from build123d import *

# Parameters (mm, degrees)
F0_R         = 12.0396
F0_R_2       = 10.7696
F1_DEPTH     = 12.065
F2_R         = 20.6121
F3_DEPTH     = 4.445
F5_DEPTH     = 16.511
F6_S5_R      = 12.0396
F6_T6_DEPTH  = 7
F6_S11_R     = 12.0396
F6_T12_DEPTH = 7
F6_S17_R     = 12.0396
F6_T18_DEPTH = 7
F6_S23_R     = 12.0396
F6_T24_DEPTH = 7
F7_W         = 10.7836972851
F7_H         = 1.905
F7_W_2       = 1.905
F7_H_2       = 10.8237928489
F7_W_3       = 10.1713027149
F7_H_3       = 10.1312071511
F8_DEPTH     = 2.54


# Not quite as in the source:
# - a fillet or chamfer that OpenCascade refuses, or shapes differently, is made with other operations: its cross-section is extruded or revolved along the edge and cut away or added


with BuildPart() as f1:
    # F0 (on Top) → F1 (new body)
    with BuildSketch(Plane.XY):
        with Locations((-31.5266512334, -46.8901731074)):
            Circle(F0_R)
        with Locations((-31.5266512334, -46.8901731074)):
            Circle(F0_R_2, mode=Mode.SUBTRACT)
    extrude(amount=F1_DEPTH)

    # F2 (on face) → F3 (join)
    with BuildSketch(Plane.XY.offset(12.065)):
        with Locations((-31.5266512334, -46.8901731074)):
            Circle(F2_R)
    extrude(amount=F3_DEPTH)

    # F4 (on face) → F5 (cut, through all)
    with BuildSketch(Plane.XY.offset(16.51)):
        with BuildLine():
            ThreePointArc((-31.7884928641, -33.1131611233), (-30.2443193797, -32.4476041714), (-29.6082253852, -30.8910624162))
            ThreePointArc((-29.6082253852, -30.8910624162), (-33.4171313906, -29.3345206609), (-31.7884928641, -33.1131611233))
        make_face()
        with BuildLine():
            ThreePointArc((-13.3019866134, -46.5860989557), (-15.5486867731, -44.3606454902), (-17.7526926267, -46.6283895083))
            ThreePointArc((-17.7526926267, -46.6283895083), (-15.5063943113, -48.8115524211), (-13.3019866134, -46.5860989557))
        make_face()
        with BuildLine():
            ThreePointArc((-28.9935999678, -62.8892183723), (-29.6606432601, -61.3004657527), (-31.2619205449, -60.6640753873))
            ThreePointArc((-31.2619205449, -60.6640753873), (-32.777664533, -64.4779709918), (-28.9935999678, -62.8892183723))
        make_face()
        with BuildLine():
            ThreePointArc((-45.3002079959, -47.1942472591), (-45.3003084592, -47.1731010282), (-45.3006098402, -47.1519567065))
            ThreePointArc((-45.3006098402, -47.1519567065), (-49.7512153901, -47.21539349), (-45.3002079959, -47.1942472591))
        make_face()
    extrude(amount=-F5_DEPTH, mode=Mode.SUBTRACT)

    # F6: chamfer of 1.905 on 4 edges, made by hand


with BuildPart() as f6_tool2:
    # F6_s3 → F6_t4 (revolve)
    with BuildSketch(Plane.XZ.offset(62.8892183723)):
        Polygon((-27.0885999678, 12.065), (-28.9935999678, 13.97), (-28.9935999678, 12.065), align=None)
    revolve(axis=Axis((-31.2191538966, -62.8892183723, 12.065), (0, 0, 1)))

    # F6_s5 → F6_t6 (cut, symmetric)
    with BuildSketch(Plane.XY.offset(13)):
        with Locations((-31.5266512334, -46.8901731074)):
            Circle(F6_S5_R)
    extrude(amount=F6_T6_DEPTH, both=True, mode=Mode.SUBTRACT)


with BuildPart() as f1_1:
    add(f1.part)

    # F6_t1: cut F6_tool2
    add(f6_tool2.part, mode=Mode.SUBTRACT)


with BuildPart() as f6_tool8:
    # F6_s9 → F6_t10 (revolve)
    with BuildSketch(Plane.XZ.offset(46.5860989557)):
        Polygon((-11.3969866134, 12.065), (-13.3019866134, 13.97), (-13.3019866134, 12.065), align=None)
    revolve(axis=Axis((-15.5275405422, -46.5860989557, 12.065), (0, 0, 1)))

    # F6_s11 → F6_t12 (cut, symmetric)
    with BuildSketch(Plane.XY.offset(13)):
        with Locations((-31.5266512334, -46.8901731074)):
            Circle(F6_S11_R)
    extrude(amount=F6_T12_DEPTH, both=True, mode=Mode.SUBTRACT)


with BuildPart() as f1_2:
    add(f1_1.part)

    # F6_t7: cut F6_tool8
    add(f6_tool8.part, mode=Mode.SUBTRACT)


with BuildPart() as f6_tool14:
    # F6_s15 → F6_t16 (revolve)
    with BuildSketch(Plane(origin=(0.8794745138, -46.2742722997, 0), x_dir=(0, 0, 1), z_dir=(0.0190022592, -0.9998194408, 0))):
        Polygon((12.065, 44.2834241002), (13.97, 46.1884241002), (12.065, 46.1884241002), align=None)
    revolve(axis=Axis((-47.5257619247, -47.1942472591, 12.065), (0, 0, 1)))

    # F6_s17 → F6_t18 (cut, symmetric)
    with BuildSketch(Plane.XY.offset(13)):
        with Locations((-31.5266512334, -46.8901731074)):
            Circle(F6_S17_R)
    extrude(amount=F6_T18_DEPTH, both=True, mode=Mode.SUBTRACT)


with BuildPart() as f1_3:
    add(f1_2.part)

    # F6_t13: cut F6_tool14
    add(f6_tool14.part, mode=Mode.SUBTRACT)


with BuildPart() as f6_tool20:
    # F6_s21 → F6_t22 (revolve)
    with BuildSketch(Plane(origin=(-32.4061257472, -0.6159008077, 0), x_dir=(0, 0, 1), z_dir=(-0.9998194408, -0.0190022592, 0))):
        Polygon((12.065, -34.4081290555), (13.97, -32.5031290555), (12.065, -32.5031290555), align=None)
    revolve(axis=Axis((-31.8307253852, -30.8910624162, 12.065), (0, 0, 1)))

    # F6_s23 → F6_t24 (cut, symmetric)
    with BuildSketch(Plane.XY.offset(13)):
        with Locations((-31.5266512334, -46.8901731074)):
            Circle(F6_S23_R)
    extrude(amount=F6_T24_DEPTH, both=True, mode=Mode.SUBTRACT)


with BuildPart() as f1_4:
    add(f1_3.part)

    # F6_t19: cut F6_tool20
    add(f6_tool20.part, mode=Mode.SUBTRACT)

    # F7 (on face) → F8 (join)
    with BuildSketch(Plane(origin=(0, 0, 12.065), x_dir=(1, 0, 0), z_dir=(0, 0, -1))):
        with Locations((-37.7473032813, 46.6444636265)):
            Rectangle(F7_W, F7_H)
        with Locations((-31.4029546387, 53.008860051)):
            Rectangle(F7_W_2, F7_H_2)
        with Locations((-31.4029546387, 46.6444636265)):
            Rectangle(F7_W_2, F7_H)
        with Locations((-25.3648032813, 46.6444636265)):
            Rectangle(F7_W_3, F7_H)
        with Locations((-31.4029546387, 40.626360051)):
            Rectangle(F7_W_2, F7_H_3)
    extrude(amount=F8_DEPTH)


solid = f1_4.part
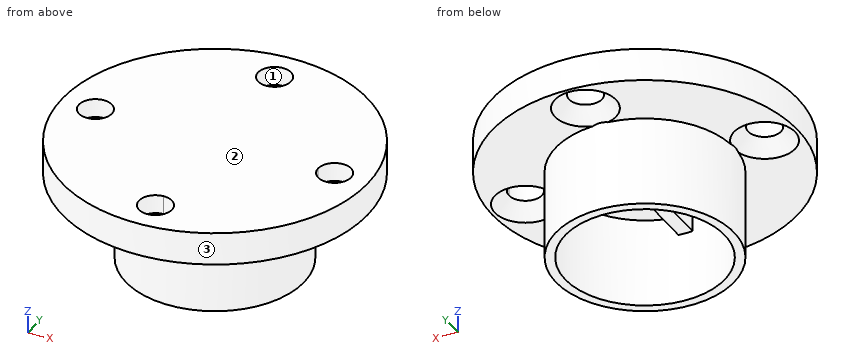
Can you work these out from the model? Positions are in its coordinate system, mm. Face numbers are marked on the shaded views. Round coordinates to 2 decimals unless told otherwise and drop trailing zeros. Order: outer loops, then holes, each group sorted by start corner. A loop starts at its lowest first (then second) coordinate and runs counter-clockwise, first axis right, second up. Notation, with made-up numbers: (83, 29.5) -> (122, 29.5) arc R24 ccw to (122, 39.5) -> close; hole circle Ø8 at (81.5, 47.25). An arc over 180 degrees is marked (long way). Write each question's results on one line, items separated by ' | '. Start each with the question number.
Item 1: If we section it at D-D, the plane z = 8.25: Write out the boundary of the cut face in (x, y), then the cut area to 3 significant figures.
Item 2: If we section it at C-C, the plane y = -39: Write out the boundary of the cut face in (x, z) (1 decimal), then the cut area to 3 significant figures.
Item 3: If we section it at A-A, the plane x = -25: Write out the boundary of the cut face in (y, z) (3 decimals), then the cut area to 3 significant figures.
Item 4: Please list where these lines run through material, in increasing order: L1, parallel to Y at x = -32, z = 4; L2, parallel to Y at x = -26, z = 11; L3, parallel to Y at x = -41, z = 11.
Item 5: If we section it at B-B, the plane z = 11.5: Write out the boundary of the cut face in (x, y).
Item 6: Thinking about a two-plate mould opening in Y: for the marked faces 1, 2 and 3, which applies, +Y half, -Y half, draft (parallel to the pull), parting line (faces both ways), or undercut?
Item 7: Will these pins go through, and if not, where does the flat tip stop? pin 1 (2.5 mm diameter, centred on x = -31.83, y = -30.89, fed in from -Z); pin 2 (3 mm diameter, centred on x = -21.5, z = 8, fed in from +Y); pin 3 (1.3 mm diameter, centred on y = -51, z = 10.5, fed in from -X); pin 4 (6 mm diameter, centred on x = -29.5, z = 11, fed in from +Y).
Results:
1) outline: circle Ø24.08 at (-31.53, -46.89); hole circle Ø21.54 at (-31.53, -46.89) | area: 91.0 mm2
2) outline: (-50.6, 12.1) -> (-40.6, 12.1) -> (-40.6, 0) -> (-38.9, 0) -> (-38.9, 12.1) -> (-32.4, 12.1) -> (-32.4, 9.5) -> (-30.5, 9.5) -> (-30.5, 12.1) -> (-24.2, 12.1) -> (-24.2, 0) -> (-22.4, 0) -> (-22.4, 12.1) -> (-12.5, 12.1) -> (-12.5, 16.5) -> (-50.6, 16.5) -> close | area: 217 mm2
3) outline: (-66.442, 12.065) -> (-57.007, 12.065) -> (-57.007, 0) -> (-55.457, 0) -> (-55.457, 12.065) -> (-47.597, 12.065) -> (-47.597, 9.525) -> (-45.692, 9.525) -> (-45.692, 12.065) -> (-38.324, 12.065) -> (-38.324, 0) -> (-36.773, 0) -> (-36.773, 12.065) -> (-27.339, 12.065) -> (-27.339, 16.51) -> (-66.442, 16.51) -> close | area: 216 mm2
4) L1: y = -58.92 to -57.65, -36.13 to -34.86 | L2: y = -57.59 to -56.13, -47.6 to -45.69, -37.65 to -36.19 | L3: y = -54.32 to -52.01, -47.6 to -45.69, -41.77 to -39.46
5) outline: circle Ø24.08 at (-31.53, -46.89); hole (-42.27, -47.6) arc R10.77 ccw to (-32.36, -57.63) -> (-32.36, -47.6) -> close; hole (-42.23, -45.69) -> (-32.36, -45.69) -> (-32.36, -36.15) arc R10.77 ccw to start; hole (-30.45, -57.61) arc R10.77 ccw to (-20.78, -47.6) -> (-30.45, -47.6) -> close; hole (-30.45, -45.69) -> (-20.82, -45.69) arc R10.77 ccw to (-30.45, -36.17) -> close
6) face 1: undercut | face 2: draft | face 3: parting line
7) pin 1: passes through | pin 2: stops at y = -38.39 | pin 3: stops at x = -43.06 | pin 4: stops at y = -26.28
